Build history of the part. All positions in model axes, mm. Face numbers are marked on the shaded views. A direction names the side the tool comes from. Give positions to 0.01 mm unless a question says otherwise; leave off trailing zeros. Order: outer loops, then holes, each group sorted by start corner. A loop starts at its lowest first (then second) coordinate and runs counter-clockwise, first axis right, second up. Notation, with made-up numbers: (85.25, 78) - (113.25, 78) arc R34 cw to (113.25, 111) - close; hole circle Ø9 at (63.25, 39). An arc over 180 degrees is marked (long way). Write each question's results on one line, items separated by ' | '. Start each with the question number.
1) Drop flat-ended pins along their axis: pin 1 Ø10 at (y, z) = (6, -9.5) entering from -X; pin 2 Ø4 at (x, z) = (14, -24.5) entering from +Y; pin 3 Ø5.5 at (x, y) = (12, -2) entering from +Z; pin 4 Ø1.9 at (x, y) = (12.5, -1.25) entering from +Z. Give the stop position or say it passes through.
2) Tool access for the marked faces 4, 5, 6 and 7: list every direction of +Z, -Z, +X, -X, +Y, -Y with a clear straight run to the whole face (end or side of a thin tool).
3) Cut at D-D on z = -1.75. List the corners of the cut face in (x, y).
4) Two-plate mould, pull along X, no slides. Class the marked faces 1, 2 and 3: +X half, -X half, draft (parallel to the pull), parting line (faces both ways), or undercut.
5) Drill centre lines: line 1 along Y through (x, z) = (4.85, -17.5); line 2 along X through (y, z) = (2.75, -24) (3 decimals); line 3 along Y through (x, z) = (4.7, -4). Where is each one in solid material? Low to high. Write a range as from..to.
6) Cut at B-B on x = -12.5. List the corners of the cut face in (y, z).
7) Cut at C-C on y = -5.25. List the corners of the cut face in (x, z) (3 decimals).
8) Cut at A-A on z = -21.5. List the corners of the cut face in (x, y) (3 decimals), plus the area to 3 significant figures.
from build123d import *

# Parameters (mm, degrees)
BOSS_EXTRUDE1_DEPTH             = 8.75
F_6_0_6_DIAMETER_HOLE1_D        = 6
TAP_DRILL_FOR_M3X0_5_TAP1_D     = 2.5
M3_CLEARANCE_HOLE1_D            = 3.2
M3_CLEARANCE_HOLE1_DEPTH        = 5
M3_CLEARANCE_HOLE1_TIP          = 0.96137699
M4_CLEARANCE_HOLE1_D            = 4.3
M4_CLEARANCE_HOLE1_DEPTH        = 4.325
M4_CLEARANCE_HOLE1_TIP          = 1.291850331
TAP_DRILL_FOR_M4X0_7_TAP1_D     = 3.3
TAP_DRILL_FOR_M4X0_7_TAP1_DEPTH = 4.325
TAP_DRILL_FOR_M4X0_7_TAP1_TIP   = 0.991420021
CUT_EXTRUDE1_DEPTH              = 31.414840202
CUT_EXTRUDE1_DEPTH_BACK         = 31.414840202
SKETCH16_W                      = 11
SKETCH16_H                      = 2.5


with BuildPart() as part:
    # Sketch1 → Boss-Extrude1 (new, symmetric)
    with BuildSketch(Plane(origin=(0, 0, 0), x_dir=(1, 0, 0), z_dir=(0, 1, 0))):
        Polygon((-7.5, 0), (7.5, 0), (7.5, 22.5), (18.5, 22.5), (18.5, 27.5), (3.175, 27.5), (3.175, 11.175), (3.175, 8), (0, 8), (-3.175, 8), (-3.175, 11.175), (-3.175, 27.5), (-18.5, 27.5), (-18.5, 22.5), (-7.5, 22.5), align=None)
    extrude(amount=BOSS_EXTRUDE1_DEPTH, both=True)

    # Ø6.0 (6) Diameter Hole1 (through all)
    with Locations(Plane.XY):
        with Locations((0, -1.25)):
            Hole(F_6_0_6_DIAMETER_HOLE1_D / 2)

    # Tap Drill for M3x0.5 Tap1 (through all)
    with Locations(Plane.ZY.offset(7.5)):
        with Locations((-4, -1.25)):
            Hole(TAP_DRILL_FOR_M3X0_5_TAP1_D / 2)

    # M3 Clearance Hole1
    with Locations(Plane.XY.offset(-22.5)):
        with Locations((12.5, -1.25), (-12.5, -1.25)):
            Hole(M3_CLEARANCE_HOLE1_D / 2, depth=M3_CLEARANCE_HOLE1_DEPTH)
            with Locations((0, 0, -(M3_CLEARANCE_HOLE1_DEPTH + M3_CLEARANCE_HOLE1_TIP / 2))):  # 118° drill point
                Cone(0, M3_CLEARANCE_HOLE1_D / 2, M3_CLEARANCE_HOLE1_TIP, mode=Mode.SUBTRACT)

    # M4 Clearance Hole1
    with Locations(Plane(origin=(7.5, 0, 0), x_dir=(0, 0, -1), z_dir=(1, 0, 0))):
        with Locations((17.5, 4.41)):
            Hole(M4_CLEARANCE_HOLE1_D / 2, depth=M4_CLEARANCE_HOLE1_DEPTH)
            with Locations((0, 0, -(M4_CLEARANCE_HOLE1_DEPTH + M4_CLEARANCE_HOLE1_TIP / 2))):  # 118° drill point
                Cone(0, M4_CLEARANCE_HOLE1_D / 2, M4_CLEARANCE_HOLE1_TIP, mode=Mode.SUBTRACT)

    # Tap Drill for M4x0.7 Tap1
    with Locations(Plane(origin=(-3.175, 0, 0), x_dir=(0, 0, -1), z_dir=(1, 0, 0))):
        with Locations((17.5, 4.41)):
            Hole(TAP_DRILL_FOR_M4X0_7_TAP1_D / 2, depth=TAP_DRILL_FOR_M4X0_7_TAP1_DEPTH)
            with Locations((0, 0, -(TAP_DRILL_FOR_M4X0_7_TAP1_DEPTH + TAP_DRILL_FOR_M4X0_7_TAP1_TIP / 2))):  # 118° drill point
                Cone(0, TAP_DRILL_FOR_M4X0_7_TAP1_D / 2, TAP_DRILL_FOR_M4X0_7_TAP1_TIP, mode=Mode.SUBTRACT)

    # Sketch16 → Cut-Extrude1 (cut, two sides: drawn at the far end of the back side and taken through both)
    with BuildSketch(Plane.XY.offset(-22.5).offset(-CUT_EXTRUDE1_DEPTH_BACK)):
        with Locations((-13, 7.5)):
            Rectangle(SKETCH16_W, SKETCH16_H)
        with Locations((13, 7.5)):
            Rectangle(SKETCH16_W, SKETCH16_H)
    extrude(amount=CUT_EXTRUDE1_DEPTH + CUT_EXTRUDE1_DEPTH_BACK, mode=Mode.SUBTRACT)


solid = part.part
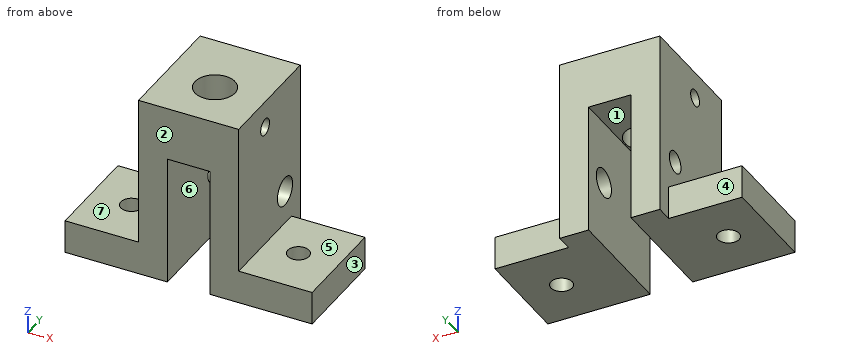
Results:
1) pin 1: x = -7.5 | pin 2: y = 6.25 | pin 3: z = -22.5 | pin 4: through
2) face 4: +Z, -Z, -X, +Y | face 5: +Z, +X, +Y, -Y | face 6: -Z, +Y, -Y | face 7: +Z, -X, +Y, -Y
3) outline: (-7.5, -8.75) - (7.5, -8.75) - (7.5, 8.75) - (-7.5, 8.75) - close; hole circle Ø6 at (0, -1.25)
4) face 1: undercut | face 2: draft | face 3: +X half
5) line 1: -8.75..2.26, 6.56..8.75 | line 2: -18.5..-3.175, 3.175..18.5 | line 3: -8.75..-2.5, 0..8.75
6) outline: (-8.75, -27.5) - (-2.85, -27.5) - (-2.85, -22.5) - (-8.75, -22.5) - close; (0.35, -27.5) - (6.25, -27.5) - (6.25, -22.5) - (0.35, -22.5) - close
7) outline: (-18.5, -27.5) - (-3.175, -27.5) - (-3.175, -8) - (3.175, -8) - (3.175, -27.5) - (18.5, -27.5) - (18.5, -22.5) - (7.5, -22.5) - (7.5, 0) - (-7.5, 0) - (-7.5, -22.5) - (-18.5, -22.5) - close
8) outline: (-7.5, -8.75) - (-3.175, -8.75) - (-3.175, 8.75) - (-7.5, 8.75) - close; (3.175, -8.75) - (7.5, -8.75) - (7.5, 8.75) - (3.175, 8.75) - close | area: 151 mm^2
